```python
from build123d import *

# Parameters (mm, degrees)
SKETCH_1_W           = 82
SKETCH_1_H           = 82
SKETCH_1_R           = 35.5
EXTRUDE_1_DEPTH      = 245
SKETCH_2_W           = 82
SKETCH_2_H           = 82
EXTRUDE_2_DEPTH      = 27
SKETCH_3_W           = 8
SKETCH_3_H           = 20
CUT_EXTRUDE_1_DEPTH  = 245
SKETCH_4_R           = 4
CUT_EXTRUDE_2_DEPTH  = 20
FILLET_2_R           = 3
FILLET_3_R           = 3
FILLET_4_R           = 3
FILLET_5_R           = 3
SKETCH_5_R           = 1.05
CUT_EXTRUDE_3_DEPTH  = 10
EXTRUDE_START        = 0.2
SKETCH_6_R           = 1.05
EXTRUDE_3_DEPTH      = 0.2
CUT_EXTRUDE_5_REACH  = 263.591
SKETCH_7_W           = 20
SKETCH_7_H           = 65
CUT_EXTRUDE_6_REACH  = 263.591
SKETCH_8_W           = 41
SKETCH_8_H           = 20
SKETCH_9_R           = 1.2
CUT_EXTRUDE_7_DEPTH  = 10
CUT_EXTRUDE_8_REACH  = 263.591
SKETCH_10_W          = 245
SKETCH_10_H          = 82
SKETCH_11_W          = 20
SKETCH_11_H          = 17
CUT_EXTRUDE_9_DEPTH  = 20
CUT_EXTRUDE_10_DEPTH = 2
SKETCH_13_W          = 21
SKETCH_13_H          = 22
CUT_EXTRUDE_11_DEPTH = 2


with BuildPart() as part:
    # 草圖1 → 填料-伸長1 (new body)
    with BuildSketch(Plane.XY):
        Rectangle(SKETCH_1_W, SKETCH_1_H)
        Circle(SKETCH_1_R, mode=Mode.SUBTRACT)
    extrude(amount=EXTRUDE_1_DEPTH)

    # 草圖2 → 填料-伸長2 (add)
    with BuildSketch(Plane(origin=(0, 0, 0), x_dir=(-1, 0, 0), z_dir=(0, 0, -1))):
        Rectangle(SKETCH_2_W, SKETCH_2_H)
    extrude(amount=EXTRUDE_2_DEPTH)

    # 草圖3 → 除料-伸長1 (cut)
    with BuildSketch(Plane.XY.offset(245)):
        with Locations((-37, 0)):
            Rectangle(SKETCH_3_W, SKETCH_3_H)
    extrude(amount=-CUT_EXTRUDE_1_DEPTH, mode=Mode.SUBTRACT)

    # 草圖4 → 除料-伸長2 (cut)
    with BuildSketch(Plane.XY.offset(245)):
        with Locations((-32.9, 33)):
            Circle(SKETCH_4_R)
        with Locations((33.1, 32.9)):
            Circle(SKETCH_4_R)
        with Locations((33, -33.1)):
            Circle(SKETCH_4_R)
        with Locations((-33, -33)):
            Circle(SKETCH_4_R)
    extrude(amount=-CUT_EXTRUDE_2_DEPTH, mode=Mode.SUBTRACT)

    # 圓角2
    fillet_2_edges = [part.edges().sort_by_distance(p)[0] for p in [
        (-36.9, 33, 225),
    ]]
    fillet(fillet_2_edges, radius=FILLET_2_R)

    # 圓角3
    fillet_3_edges = [part.edges().sort_by_distance(p)[0] for p in [
        (29.1, 32.9, 225),
    ]]
    fillet(fillet_3_edges, radius=FILLET_3_R)

    # 圓角4
    fillet_4_edges = [part.edges().sort_by_distance(p)[0] for p in [
        (-37, -33, 225),
    ]]
    fillet(fillet_4_edges, radius=FILLET_4_R)

    # 圓角5
    fillet_5_edges = [part.edges().sort_by_distance(p)[0] for p in [
        (29, -33.1, 225),
    ]]
    fillet(fillet_5_edges, radius=FILLET_5_R)

    # 草圖5 → 除料-伸長3 (cut)
    with BuildSketch(Plane(origin=(0, 41, 0), x_dir=(1, 0, 0), z_dir=(0, 1, 0))):
        with Locations(Location((-36.75, 22.75, 0), (0, 0, 270))):
            Circle(SKETCH_5_R)
        with Locations(Location((-36.75, 4.75, 0), (0, 0, 270))):
            Circle(SKETCH_5_R)
    extrude(amount=-CUT_EXTRUDE_3_DEPTH, mode=Mode.SUBTRACT)

    # 草圖6 → 填料-伸長3 (add)
    with BuildSketch(Plane(origin=(0, 35, 0), x_dir=(1, 0, 0), z_dir=(0, 1, 0)).offset(EXTRUDE_START)):
        with Locations(Location((-36.75, 22.75, 0), (0, 0, 270))):
            Circle(SKETCH_6_R)
        with Locations(Location((-36.75, 4.75, 0), (0, 0, 270))):
            Circle(SKETCH_6_R)
    extrude(amount=-EXTRUDE_3_DEPTH)

    # 草圖7 → 除料-伸長5 (cut, up to next)
    with BuildSketch(Plane(origin=(-41, 0, 0), x_dir=(0, 0, -1), z_dir=(1, 0, 0)), mode=Mode.PRIVATE) as cut_extrude_5_sk1:
        with Locations((17, -8.5)):
            Rectangle(SKETCH_7_W, SKETCH_7_H)
    cut_extrude_5_tool1 = extrude(cut_extrude_5_sk1.sketch, amount=CUT_EXTRUDE_5_REACH, mode=Mode.PRIVATE) & part.part
    add(cut_extrude_5_tool1.solids().sort_by_distance((-41, -8.5, -17))[0], mode=Mode.SUBTRACT)

    # 草圖8 → 除料-伸長6 (cut, up to next)
    with BuildSketch(Plane(origin=(0, 41, 0), x_dir=(1, 0, 0), z_dir=(0, 1, 0)), mode=Mode.PRIVATE) as cut_extrude_6_sk1:
        with Locations((20.5, 17)):
            Rectangle(SKETCH_8_W, SKETCH_8_H)
    cut_extrude_6_tool1 = extrude(cut_extrude_6_sk1.sketch, amount=-CUT_EXTRUDE_6_REACH, mode=Mode.PRIVATE) & part.part
    add(cut_extrude_6_tool1.solids().sort_by_distance((20.5, 41, -17))[0], mode=Mode.SUBTRACT)

    # 草圖9 → 除料-伸長7 (cut)
    with BuildSketch(Plane(origin=(0, 0, -7), x_dir=(-1, 0, 0), z_dir=(0, 0, -1))):
        with Locations((-33, 33)):
            Circle(SKETCH_9_R)
        with Locations((-33, -33)):
            Circle(SKETCH_9_R)
        with Locations((33, -33)):
            Circle(SKETCH_9_R)
        with Locations((36, 20)):
            Circle(SKETCH_9_R)
    extrude(amount=-CUT_EXTRUDE_7_DEPTH, mode=Mode.SUBTRACT)

    # 草圖10 → 除料-伸長8 (cut, up to next)
    with BuildSketch(Plane.ZY.offset(41), mode=Mode.PRIVATE) as cut_extrude_8_sk1:
        with Locations((122.5, 0)):
            Rectangle(SKETCH_10_W, SKETCH_10_H)
    cut_extrude_8_tool1 = extrude(cut_extrude_8_sk1.sketch, amount=-CUT_EXTRUDE_8_REACH, mode=Mode.PRIVATE) & part.part
    add(cut_extrude_8_tool1.solids().sort_by_distance((-41, 0, 122.5))[0], mode=Mode.SUBTRACT)

    # 草圖11 → 除料-伸長9 (cut)
    with BuildSketch(Plane(origin=(0, 0, 0), x_dir=(0, 0, -1), z_dir=(1, 0, 0))):
        with Locations((17, 32.5)):
            Rectangle(SKETCH_11_W, SKETCH_11_H)
    extrude(amount=-CUT_EXTRUDE_9_DEPTH, mode=Mode.SUBTRACT)

    # 草圖12 → 除料-伸長10 (cut)
    with BuildSketch(Plane(origin=(0, 0, -7), x_dir=(-1, 0, 0), z_dir=(0, 0, -1))):
        Polygon((20, 41), (20, 24), (41, 24), (41, -41), (-41, -41), (-41, 41), align=None)
    extrude(amount=-CUT_EXTRUDE_10_DEPTH, mode=Mode.SUBTRACT)

    # 草圖13 → 除料-伸長11 (cut)
    with BuildSketch(Plane.XZ.offset(-24)):
        with Locations((-30.5, -16)):
            Rectangle(SKETCH_13_W, SKETCH_13_H)
    extrude(amount=-CUT_EXTRUDE_11_DEPTH, mode=Mode.SUBTRACT)


solid = part.part
```
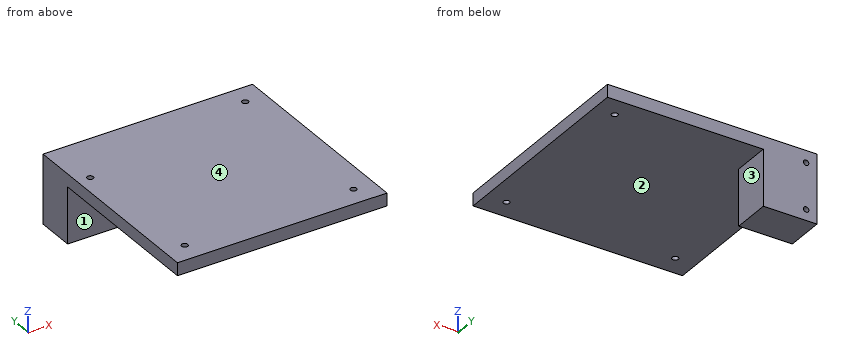
Part model, mm, in its own coordinate system. Face numbers are marked on the shaded views. A direction names the side the tool comes from. Give positions to 0.01 mm unless a question says otherwise; leave off trailing zeros. Order: outer loops, then holes, each group sorted by start corner. A loop starts at its lowest first (then second) coordinate and runs counter-clockwise, first axis right, second up. Notation, with made-up numbers: M -8.75,80.5 L 27.25,80.5 A27 cw 27.25,106.5 Z; hole C 22.25,-3.5 d5. An arc over 180 degrees is marked long. Use a Markdown table: item, result. Add a question column.
(1) Saw through at D-D, the plane x = -23. Give the cut face in (y, z), and give its area (3 significant figures).
(2) Drop flat-ended pins along their axis: P1, Ø1, axis at x = -36.5, z = -5, coming from the +Y side; P2, Ø12, axis at y = 26, z = -18, coming from the +X side; P3, Ø1.9, axis at x = 33, y = -33, coming from the -Z side; P4, Ø3, axis at x = -19.5, y = -19.5, coming from the -Z side. Give the stop position or say it passes through.
(3) Saw through at B-B, the plane x = 33. Give the cut face in (y, z), and give its area (3 significant figures).
(4) 3-axis set-ups, long thin cutter, end or side, ignore diameter. For the marked faces 1, 2, 3 and 4: which of +Z, -Z, +X, -X, +Y, -Y reach the whole face in a straight line?
(5) Saw through at C-C, the plane z = -22.75. Give the cut face in (x, y), and give its area (3 significant figures).
(6) Saw through at A-A, the plane y = 33. Give the cut face in (x, z).
(7) Probe line 1 along Y through (x, z) = (-33, -3.55); line 2 along X through (y, z) = (33.15, -22.75); line 3 along X through (y, z) = (38.25, -4.75). List the from-to ranges inside material, lowest first. Write a range as [from, to].
Answer key:
| question | item | result |
|---|---|---|
| 1 | outline | M -41,-5 L 26,-5 L 26,-27 L 41,-27 L 41,0 L -41,0 Z |
| 1 | area | 740 mm^2 |
| 2 | P1 | y = 35.2 |
| 2 | P2 | x = -20 |
| 2 | P3 | through |
| 2 | P4 | z = -5 |
| 3 | outline | M -41,-5 L -34.2,-5 L -34.2,0 L -41,0 Z; M -31.8,-5 L 31.8,-5 L 31.8,0 L -31.8,0 Z; M 34.2,-5 L 41,-5 L 41,0 L 34.2,0 Z |
| 3 | area | 386 mm^2 |
| 4 | face 1 | -Z, +X, -X, -Y |
| 4 | face 2 | -Z, +X, -Y |
| 4 | face 3 | -Z, +X, +Y, -Y |
| 4 | face 4 | +Z, +X, -X, +Y, -Y |
| 5 | outline | M -41,26 L -20,26 L -20,41 L -35.7,41 L -35.7,35.2 L -37.8,35.2 L -37.8,41 L -41,41 Z; hole M -37.8,31 L -35.7,31 L -35.7,35 L -37.8,35 Z |
| 5 | area | 294 mm^2 |
| 6 | outline | M -41,-27 L -20,-27 L -20,-5 L 31.8,-5 L 31.8,0 L -41,0 Z; M 34.2,-5 L 41,-5 L 41,0 L 34.2,0 Z; hole C -36.75,-22.75 d2.1; hole C -36.75,-4.75 d2.1 |
| 7 | line 1 | [-41, -34.2], [-31.8, 41] |
| 7 | line 2 | [-41, -37.8], [-35.7, -20] |
| 7 | line 3 | [-41, -37.8], [-35.7, 41] |
